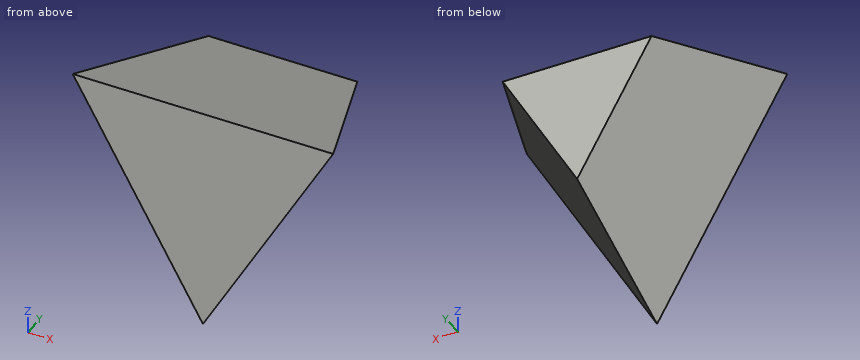
```python
from build123d import *

# Parameters (mm, degrees)
BOSS_EXTRUDE1_DEPTH = 101.6
SKETCH3_W           = 415.71343084
SKETCH3_H           = 232.25163297
CUT_EXTRUDE1_DEPTH  = 152.4
SKETCH4_W           = 330.261627224
SKETCH4_H           = 257.519114475
CUT_EXTRUDE2_DEPTH  = 152.4
SKETCH5_W           = 304.13342749
SKETCH5_H           = 210.120003228
CUT_EXTRUDE3_DEPTH  = 152.4


with BuildPart() as part:
    # Sketch1 → Boss-Extrude1 (new body)
    with BuildSketch(Plane(origin=(0, 0, 0), x_dir=(1, 0, 0), z_dir=(0, 1, 0))):
        Polygon((0, 102.652877862), (-88.9, -51.326438931), (88.9, -51.326438931), align=None)
    extrude(amount=BOSS_EXTRUDE1_DEPTH)

    # Sketch3 → Cut-Extrude1 (cut)
    with BuildSketch(Plane(origin=(-42.459701493, 10.614925373, -24.514120086), x_dir=(0.4832445480711858, -0.0803381317273392, -0.8717915412241828), z_dir=(0.846414739030318, -0.2116036847575797, 0.4886777774252209))):
        with Locations((15.518535429, 25.810339784)):
            Rectangle(SKETCH3_W, SKETCH3_H)
    extrude(amount=-CUT_EXTRUDE1_DEPTH, mode=Mode.SUBTRACT)

    # Sketch4 → Cut-Extrude2 (cut)
    with BuildSketch(Plane(origin=(0, 10.614925373, 49.028240173), x_dir=(-1, 0, 0), z_dir=(0, -0.2116036847575795, -0.9773555548504419))):
        with Locations((6.792319927, 42.566259276)):
            Rectangle(SKETCH4_W, SKETCH4_H)
    extrude(amount=-CUT_EXTRUDE2_DEPTH, mode=Mode.SUBTRACT)

    # Sketch5 → Cut-Extrude3 (cut)
    with BuildSketch(Plane(origin=(42.459701493, 10.614925373, -24.514120086), x_dir=(0.4832445480711859, 0.08033813172733906, 0.8717915412241828), z_dir=(-0.8464147390303179, -0.21160368475757932, 0.4886777774252209))):
        with Locations((15.433156883, 49.391097897)):
            Rectangle(SKETCH5_W, SKETCH5_H)
    extrude(amount=-CUT_EXTRUDE3_DEPTH, mode=Mode.SUBTRACT)


solid = part.part
```
Geometry: final body of the model. Coordinates: model frame, mm. Round coordinates to 2 decimals unless told otherwise and drop trailing zeros. Order: outer loops, then holes, each group sorted by start corner. A loop starts at its lowest first (then second) coordinate and runs counter-clockwise, first axis right, second up. Notation, with made-up numbers: M -18.75,47 L 39.25,47 A29 cw 39.25,75 Z; hole C 60,49 d11. An arc over 180 degrees is marked long. One line per item, written item: value.
(1) Cut plane A-A (x = 10). Return the cut outline in (y, z), and give its area (3 significant figures).
Result sheet:
outline: M 0,-85.33 L 101.6,-41.34 L 101.6,29.33 L 0,51.33 Z
area: 10,500 mm2
(2) Cut plane C-C (z = 35.5). Return the cut outline in (x, y), and give its area (3 significant figures).
Result sheet:
outline: M -79.76,0 L 79.76,0 L 61.49,73.1 L -61.49,73.1 Z
area: 10,300 mm2
(3) Pin query (flat end, axial travel): P1, Ø10, axis at y = 66, z = -50.5, coming from the +X side; P2, Ø2, axis at y = 17, z = -81.5, coming from the -X side; P3, Ø10, axis at x = 31, y = 44, coming from the +Z side. Return the tip coordinate at first contact, or that it passes through.
Result sheet:
P1: x = 16.76
P2: x = -8.59
P3: z = 42.88
(4) Line query: probe 1 along X at (y, z) = (38.5, -52); probe 2 along Z at (x, y) = (30, 57); probe 3 along X at (y, z) = (96, -7). Output: solid intervals per line, ascending. Write a range as [from, to].
Result sheet:
probe 1: [-19.62, 19.62]
probe 2: [-26.01, 38.99]
probe 3: [-31.23, 31.23]
(5) Cut plane D-D (y = 26). Return the cut outline in (x, z), and give its area (3 significant figures).
Result sheet:
outline: M -79.15,45.7 L 0,-91.39 L 79.15,45.7 Z
area: 10,900 mm2
(6) Cut plane B-B (y = 36.5). Return the cut outline in (x, z).
Result sheet:
outline: M -75.21,43.42 L 0,-86.85 L 75.21,43.42 Z
